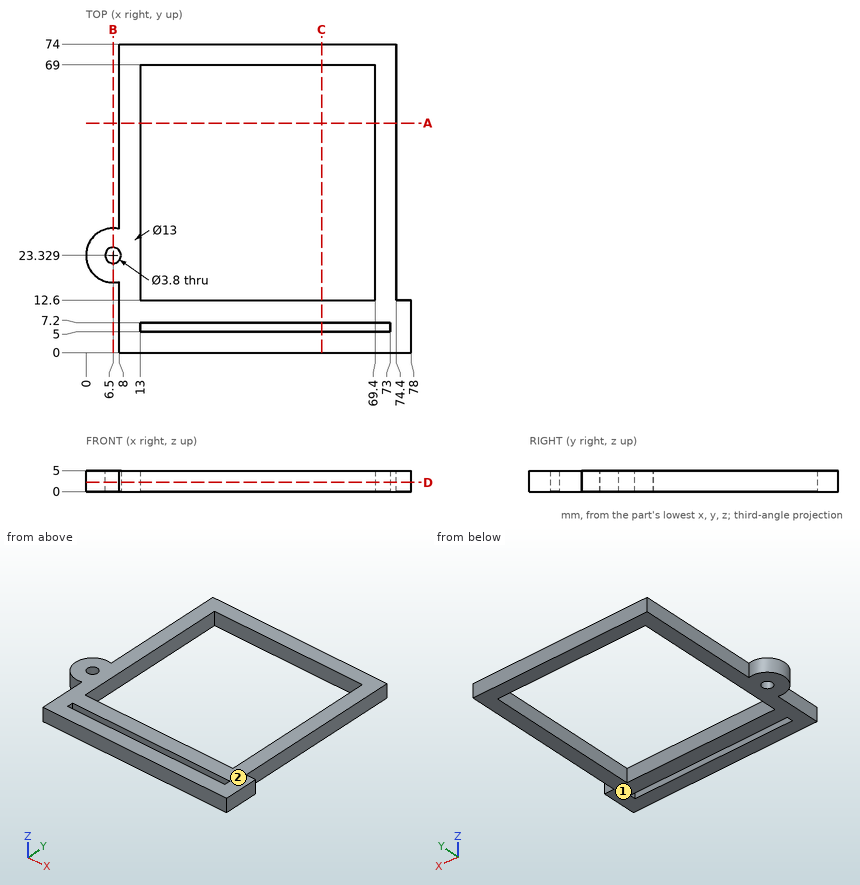
Part print with two shaded views. Sizes in mm from the minimum x, y, z corner. Give positions to 0.01 mm unless a question says otherwise; leave off trailing zeros. Order: outer loops, then holes, each group sorted by start corner. A loop starts at its lowest first (then second) coordinate and runs counter-clockwise, first axis right, second up.
1) Saw through at B-B, the plane x = 6.5. Write the cut outline in (y, z).
2) Wall check: probe 1 along Y at (x, z) = (17.5, 3.05); probe 2 along X at (y, z) = (35, 2.4); probe 3 along Y at (x, z) = (6.5, 3.85). Give the ranges that are in metal, low to high.
3) Saw through at D-D, the plane z = 2.2. Write the cut outline in (x, y).
4) Mould opens along Z. For the marked faces 1 and 2 say: +Z half, -Z half, draft (parallel to the pull), parting line (faces both ways), or undercut.
5) Saw through at A-A, the plane y = 55. Write the cut outline in (x, z), then the cut area to 3 significant figures.
6) Saw through at C-C, the plane x = 56.5. Write the cut outline in (y, z), then the cut area to 3 significant figures.
7) Pin check, flat tips, straight feed: pin 1 (2.5 mm diameter, centred on y = 49.5, z = 1.5, fed in from -X); pin 2 (1.8 mm diameter, centred on x = 76, z = 3.5, fed in from +Y). Stop position of each tip, or through.
Computed:
1. outline: (16.83, 0) - (21.43, 0) - (21.43, 5) - (16.83, 5) - close; (25.23, 0) - (29.83, 0) - (29.83, 5) - (25.23, 5) - close
2. probe 1: y = 0 to 5, 7.2 to 12.6, 69 to 74
2. probe 2: x = 8 to 13, 69.4 to 74.4
2. probe 3: y = 16.83 to 21.43, 25.23 to 29.83
3. outline: (8, 0) - (78, 0) - (78, 12.6) - (74.4, 12.6) - (74.4, 74) - (8, 74) - (8, 29.65) arc R6.5 ccw (long way) to (8, 17) - close; hole circle Ø3.8 at (6.5, 23.33); hole (13, 5) - (73, 5) - (73, 7.2) - (13, 7.2) - close; hole (13, 12.6) - (69.4, 12.6) - (69.4, 69) - (13, 69) - close
4. face 1: -Z half
4. face 2: +Z half
5. outline: (8, 0) - (13, 0) - (13, 5) - (8, 5) - close; (69.4, 0) - (74.4, 0) - (74.4, 5) - (69.4, 5) - close
5. area: 50.0 mm2
6. outline: (0, 0) - (5, 0) - (5, 5) - (0, 5) - close; (7.2, 0) - (12.6, 0) - (12.6, 5) - (7.2, 5) - close; (69, 0) - (74, 0) - (74, 5) - (69, 5) - close
6. area: 77.0 mm2
7. pin 1: stops at x = 8
7. pin 2: stops at y = 12.6
